from build123d import *

# Parameters (mm, degrees)
F1_DEPTH = 5
F2_DEPTH = 15
F0_R     = 10
F3_DEPTH = 20
F4_DEPTH = 30
F5_SIZE  = 1


with BuildPart() as f1:
    # F0 (on Front) → F1 (new body)
    with BuildSketch(Plane.XZ):
        with BuildLine():
            Line((40, 139.3735986477), (40, 165.2271164186))
            ThreePointArc((40, 165.2271164186), (0, 170), (-40, 165.2271164186))
            Line((-40, 165.2271164186), (-40, 139.3735986477))
            ThreePointArc((-40, 139.3735986477), (0, 145), (40, 139.3735986477))
        make_face()
        with BuildLine():
            Line((-40, 139.3735986477), (-40, 165.2271164186))
            ThreePointArc((-40, 165.2271164186), (-170, 0), (-40, -165.2271164186))
            Line((-40, -165.2271164186), (-40, -139.3735986477))
            ThreePointArc((-40, -139.3735986477), (-145, 0), (-40, 139.3735986477))
        make_face()
        with BuildLine():
            ThreePointArc((-40, -165.2271164186), (0, -170), (40, -165.2271164186))
            Line((40, -165.2271164186), (40, -139.3735986477))
            ThreePointArc((40, -139.3735986477), (0, -145), (-40, -139.3735986477))
            Line((-40, -139.3735986477), (-40, -165.2271164186))
        make_face()
        with BuildLine():
            ThreePointArc((40, -165.2271164186), (133.6038921589, -105.1189802081), (170, 0))
            ThreePointArc((170, 0), (133.6038921589, 105.1189802081), (40, 165.2271164186))
            Line((40, 165.2271164186), (40, 139.3735986477))
            ThreePointArc((40, 139.3735986477), (115.812348219, 87.2496418331), (145, 0))
            ThreePointArc((145, 0), (115.812348219, -87.2496418331), (40, -139.3735986477))
            Line((40, -139.3735986477), (40, -165.2271164186))
        make_face()
    extrude(amount=F1_DEPTH)

    # F0 (on Front) → F2 (join)
    with BuildSketch(Plane.XZ):
        with BuildLine():
            Line((40, 122.6417547167), (40, 139.3735986477))
            ThreePointArc((40, 139.3735986477), (0, 145), (-40, 139.3735986477))
            Line((-40, 139.3735986477), (-40, 122.6417547167))
            ThreePointArc((-40, 122.6417547167), (0, 129), (40, 122.6417547167))
        make_face()
        with BuildLine():
            Line((-40, 122.6417547167), (-40, 139.3735986477))
            ThreePointArc((-40, 139.3735986477), (-145, 0), (-40, -139.3735986477))
            Line((-40, -139.3735986477), (-40, -122.6417547167))
            ThreePointArc((-40, -122.6417547167), (-129, 0), (-40, 122.6417547167))
        make_face()
        with BuildLine():
            ThreePointArc((-40, -139.3735986477), (0, -145), (40, -139.3735986477))
            Line((40, -139.3735986477), (40, -122.6417547167))
            ThreePointArc((40, -122.6417547167), (0, -129), (-40, -122.6417547167))
            Line((-40, -122.6417547167), (-40, -139.3735986477))
        make_face()
        with BuildLine():
            ThreePointArc((145, 0), (115.812348219, 87.2496418331), (40, 139.3735986477))
            Line((40, 139.3735986477), (40, 122.6417547167))
            ThreePointArc((40, 122.6417547167), (104.4054596274, 75.7660874006), (129, 0))
            ThreePointArc((129, 0), (104.4054596274, -75.7660874006), (40, -122.6417547167))
            Line((40, -122.6417547167), (40, -139.3735986477))
            ThreePointArc((40, -139.3735986477), (115.812348219, -87.2496418331), (145, 0))
        make_face()
    extrude(amount=F2_DEPTH)

    # F0 (on Front) → F3 (join)
    with BuildSketch(Plane.XZ):
        with BuildLine():
            Line((40, -122.6417547167), (40, 122.6417547167))
            ThreePointArc((40, 122.6417547167), (0, 129), (-40, 122.6417547167))
            Line((-40, 122.6417547167), (-40, -122.6417547167))
            ThreePointArc((-40, -122.6417547167), (0, -129), (40, -122.6417547167))
        make_face()
        Circle(F0_R, mode=Mode.SUBTRACT)
    extrude(amount=F3_DEPTH)

    # F0 (on Front) → F4 (cut)
    with BuildSketch(Plane.XZ):
        with BuildLine():
            ThreePointArc((40, -165.2271164186), (133.6038921589, -105.1189802081), (170, 0))
            ThreePointArc((170, 0), (133.6038921589, 105.1189802081), (40, 165.2271164186))
            Line((40, 165.2271164186), (40, 139.3735986477))
            ThreePointArc((40, 139.3735986477), (115.812348219, 87.2496418331), (145, 0))
            ThreePointArc((145, 0), (115.812348219, -87.2496418331), (40, -139.3735986477))
            Line((40, -139.3735986477), (40, -165.2271164186))
        make_face()
        with BuildLine():
            Line((-40, 139.3735986477), (-40, 165.2271164186))
            ThreePointArc((-40, 165.2271164186), (-170, 0), (-40, -165.2271164186))
            Line((-40, -165.2271164186), (-40, -139.3735986477))
            ThreePointArc((-40, -139.3735986477), (-145, 0), (-40, 139.3735986477))
        make_face()
        with BuildLine():
            ThreePointArc((145, 0), (115.812348219, 87.2496418331), (40, 139.3735986477))
            Line((40, 139.3735986477), (40, 122.6417547167))
            ThreePointArc((40, 122.6417547167), (104.4054596274, 75.7660874006), (129, 0))
            ThreePointArc((129, 0), (104.4054596274, -75.7660874006), (40, -122.6417547167))
            Line((40, -122.6417547167), (40, -139.3735986477))
            ThreePointArc((40, -139.3735986477), (115.812348219, -87.2496418331), (145, 0))
        make_face()
        with BuildLine():
            Line((-40, 122.6417547167), (-40, 139.3735986477))
            ThreePointArc((-40, 139.3735986477), (-145, 0), (-40, -139.3735986477))
            Line((-40, -139.3735986477), (-40, -122.6417547167))
            ThreePointArc((-40, -122.6417547167), (-129, 0), (-40, 122.6417547167))
        make_face()
        with BuildLine():
            ThreePointArc((129, 0), (104.4054596274, 75.7660874006), (40, 122.6417547167))
            Line((40, 122.6417547167), (40, -122.6417547167))
            ThreePointArc((40, -122.6417547167), (104.4054596274, -75.7660874006), (129, 0))
        make_face()
    extrude(amount=F4_DEPTH, mode=Mode.SUBTRACT)

    # F5
    f5_edges = [f1.edges().sort_by_distance(p)[0] for p in [
        (0, -20, -129),
        (0, -15, -145),
        (0, -15, 145),
        (0, -5, 170),
        (0, -5, -170),
        (0, -20, 129),
    ]]
    chamfer(f5_edges, length=F5_SIZE)


solid = f1.part
Geometry: final body of the model. Coordinates: model frame, mm. A direction names the side the tool comes from. Round coordinates to 2 decimals unless told otherwise and drop trailing zeros. Loops run counter-clockwise (first coordinate to the right, second up) from the corner with the lowest first, then second, coordinate; pieces in that order, holes last. Notation, with made-up numbers: M 10.5,84 L 66.5,84 A29 cw 66.5,120 Z; hole C -37,45 d7. An arc over 180 degrees is marked long. One line per question, with ' | ' between items.
(1) Cut plane C-C on y = -11. Return the cut outline in (x, z), plus the area to 3 significant figures.
Check result:
outline: M -40,-139.37 A145 ccw 40,-139.37 L 40,139.37 A145 ccw -40,139.37 Z; hole C 0,0 d20 | area: 22,600 mm2
(2) Cut plane B-B on z = 0. Return the cut outline in (x, y).
Check result:
outline: M -40,-20 L -10,-20 L -10,0 L -40,0 Z; M 10,-20 L 40,-20 L 40,0 L 10,0 Z
(3) Access query for faces 1 (the cylindrical face through (0.6, -17, 129)), 2 (the cylindrical face through (-0.6, -17, -129)), 3 (the flat face through (17, -20, 2)). Directions: +Z, -Z, +X, -X, +Y, -Y. A direction counts if a zero-diameter tool reaches every point of the face in a straight line with its end or side. Return the directions, or none.
Check result:
face 1: +Z, -Y | face 2: -Z, -Y | face 3: +Z, -Z, +X, -X, -Y
(4) Contact query for flat-ended pins moving along their axis: P1, Ø4, axis at x = -1.5, y = -18, coming from the +Z side; P2, Ø1.5, axis at x = -17.5, y = -11.5, coming from the +Z side; P3, Ø6.5, axis at x = 16.5, z = 132.5, coming from the -Y side. Output: stop coordinate, or through.
Check result:
P1: stops at z = 129 | P2: stops at z = 144.03 | P3: stops at y = -15
(5) Cut plane A-A on x = 0. Return the cut outline in (y, z), plus the area to 3 significant figures.
Check result:
outline: M -20,-128 L -19,-129 L -15,-129 L -15,-144 L -14,-145 L -5,-145 L -5,-169 L -4,-170 L 0,-170 L 0,-10 L -20,-10 Z; M -20,10 L 0,10 L 0,170 L -4,170 L -5,169 L -5,145 L -14,145 L -15,144 L -15,129 L -19,129 L -20,128 Z | area: 5,490 mm2
(6) Material intervals for line 1 along Z through (x, y) = (0, -9.25); line 2 along Z through (x, y) = (0, -15.75); line 3 along Y through (x, z) = (27, 136.5), sorted ascending. Write a range as from..to.
Check result:
line 1: z = -145..-10, 10..145 | line 2: z = -129..-10, 10..129 | line 3: y = -15..0
